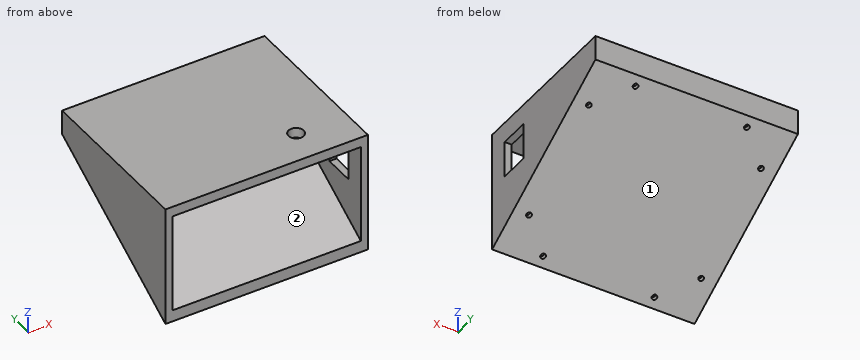
from build123d import *

# Parameters (mm, degrees)
BOSS_EXTRUDE1_DEPTH      = 200
SHELL1_T                 = -10
SHELL1_THICKNESS_2_DEPTH = 3
SHELL1_THICKNESS_3_DEPTH = 3
SKETCH4_R                = 2.5
CUT_EXTRUDE2_DEPTH       = 5
SKETCH5_W                = 36
SKETCH5_H                = 30
CUT_EXTRUDE3_DEPTH       = 20
SKETCH6_R                = 7.5
CUT_EXTRUDE4_DEPTH       = 20


with BuildPart() as part:
    # Sketch2 → Boss-Extrude1 (new body)
    with BuildSketch(Plane(origin=(0, 0, 0), x_dir=(0, 0, -1), z_dir=(1, 0, 0))):
        Polygon((0, 60.789473684), (24.5, 60.789473684), (119.5, -103.755353035), (0, -103.755353035), align=None)
    extrude(amount=BOSS_EXTRUDE1_DEPTH)

    # Shell1
    shell1_openings = [part.faces().sort_by_distance(p)[0] for p in [
        (100, -103.755353035, -59.75),
    ]]
    offset(amount=SHELL1_T, openings=shell1_openings, kind=Kind.INTERSECTION)

    # Shell1 thickness 2 face (on inner face of the shell) → Shell1 thickness 2 (cut)
    with BuildSketch(Plane(origin=(190, -48.02643305, -42.888943831), x_dir=(0, 0, 1), z_dir=(1, 0, 0))):
        Polygon((32.888943831, -98.815906734), (24.162446523, -98.815906734), (-65.064050785, 55.728919985), (32.888943831, 55.728919985), align=None)
    extrude(amount=SHELL1_THICKNESS_2_DEPTH, mode=Mode.SUBTRACT)

    # Shell1 thickness 3 face (on inner face of the shell) → Shell1 thickness 3 (cut)
    with BuildSketch(Plane(origin=(10, -48.02643305, -42.888943831), x_dir=(0, 0, -1), z_dir=(-1, 0, 0))):
        Polygon((-24.162446523, -98.815906734), (-32.888943831, -98.815906734), (-32.888943831, 55.728919985), (65.064050785, 55.728919985), align=None)
    extrude(amount=SHELL1_THICKNESS_3_DEPTH, mode=Mode.SUBTRACT)

    # Sketch4 → Cut-Extrude2 (cut)
    with BuildSketch(Plane(origin=(0, 25.806179617, -44.697614247), x_dir=(-1, 0, 0), z_dir=(0, 0.499999999999998, -0.8660254037844397))):
        with Locations(Location((-185, 0.395228493, 0), (0, 0, 90))):
            Circle(SKETCH4_R)
        with Locations(Location((-185, -109.604771507, 0), (0, 0, 90))):
            Circle(SKETCH4_R)
        with Locations(Location((-155, -139.604771507, 0), (0, 0, 90))):
            Circle(SKETCH4_R)
        with Locations(Location((-45, -139.604771507, 0), (0, 0, 90))):
            Circle(SKETCH4_R)
        with Locations(Location((-15, -109.604771507, 0), (0, 0, 90))):
            Circle(SKETCH4_R)
        with Locations(Location((-15, 0.395228493, 0), (0, 0, 90))):
            Circle(SKETCH4_R)
        with Locations(Location((-45, 30.395228493, 0), (0, 0, 90))):
            Circle(SKETCH4_R)
        with Locations(Location((-155, 30.395228493, 0), (0, 0, 90))):
            Circle(SKETCH4_R)
    extrude(amount=-CUT_EXTRUDE2_DEPTH, mode=Mode.SUBTRACT)

    # Sketch5 → Cut-Extrude3 (cut)
    with BuildSketch(Plane(origin=(200, 0, 0), x_dir=(0, 0, -1), z_dir=(1, 0, 0))):
        with Locations((38, -68.755353035)):
            Rectangle(SKETCH5_W, SKETCH5_H)
    extrude(amount=-CUT_EXTRUDE3_DEPTH, mode=Mode.SUBTRACT)

    # Sketch6 → Cut-Extrude4 (cut)
    with BuildSketch(Plane.XY):
        with Locations((150, -70.035876083)):
            Circle(SKETCH6_R)
    extrude(amount=-CUT_EXTRUDE4_DEPTH, mode=Mode.SUBTRACT)


solid = part.part
For this review, take the finished solid that the model builds, in its own axes (mm). Face numbers are marked on the shaded views. A direction names the side the tool comes from. Round coordinates to 2 decimals unless told otherwise and drop trailing zeros. Order: outer loops, then holes, each group sorted by start corner. A loop starts at its lowest first (then second) coordinate and runs counter-clockwise, first axis right, second up. Notation, with made-up numbers: M 33.25,55 L 88.25,55 A22 ccw 88.25,84 Z; hole C -1.75,51 d1. An arc over 180 degrees is marked long. Use a Markdown table: item, result. Add a question column.
Item 1: Add section C-C, the plane x = 82. Give the boundary of the cut face in (y, z), then the cut area to 3 significant figures.
Item 2: Add section B-B, the plane y = 15. Give the boundary of the cut face in (x, z), then the cut area to 3 significant figures.
Item 3: To check wall thickness, follow line 1 along Y through (x, z) = (150, -2); line 2 along X through (y, z) = (-20.5, -12.5); line 3 along Z through (x, y) = (62, -83). State the ranges of each line that lie inside material, in increasing order.
Item 4: Add section A-A, the plane x = 150. Give the boundary of the cut face in (y, z), then the cut area to 3 significant figures.
Item 5: Insertion check: pin 1 (7 mm diameter, centred on x = 85, z = -12.5, fed in from -Y); pin 2 (2 mm diameter, centred on x = 197.5, y = -63, fed in from -Z); pin 3 (4 mm diameter, centred on x = 64.5, z = -106, fed in from +Y); pin 4 (12 mm diameter, centred on x = 164.5, z = -77.5, fed in from +Y). Each pin has a flat end and moves straight along its axis. Give the tip position at first contact, or say it passes through.
Item 6: Add section D-D, the plane y = -35. Give the boundary of the cut face in (x, z), then the cut area to 4 significant figures.
Item 7: Tool access review of the marked faces 1 and 2: name each direction out of +Z, -Z, +X, -X, +Y, -Y from which nothing blocks a thin tool from reaching the whole face with its end or side.
Geometry results:
| question | item | result |
|---|---|---|
| 1 | outline | M -103.76,-119.5 L 60.79,-24.5 L 60.79,0 L -103.76,0 L -103.76,-10 L 50.79,-10 L 50.79,-18.73 L -103.76,-107.95 Z |
| 1 | area | 3,600 mm² |
| 2 | outline | M 0,-50.94 L 200,-50.94 L 200,0 L 0,0 Z; hole M 7,-39.39 L 193,-39.39 L 193,-10 L 7,-10 Z |
| 2 | area | 4,720 mm² |
| 3 | line 1 | y = -103.76 to -77.54, -62.54 to 60.79 |
| 3 | line 2 | x = 0 to 7, 193 to 200 |
| 3 | line 3 | z = -107.52 to -95.97, -10 to 0 |
| 4 | outline | M -103.76,-119.5 L 60.79,-24.5 L 60.79,0 L -62.54,0 L -62.54,-10 L 50.79,-10 L 50.79,-18.73 L -103.76,-107.95 Z; M -103.76,-10 L -77.54,-10 L -77.54,0 L -103.76,0 Z |
| 4 | area | 3,450 mm² |
| 5 | pin 1 | stops at y = -103.76 |
| 5 | pin 2 | stops at z = -96.55 |
| 5 | pin 3 | stops at y = -76.91 |
| 5 | pin 4 | stops at y = -20.62 |
| 6 | outline | M 0,-79.8 L 200,-79.8 L 200,0 L 0,0 Z; hole M 7,-68.26 L 193,-68.26 L 193,-10 L 7,-10 Z |
| 6 | area | 5,125 mm² |
| 7 | face 1 | -Z, +X, -X, +Y |
| 7 | face 2 | -Y |
